Read the model definition and answer for the solid it produces. Units are mm, in the model's axes. Face numbers are marked on the shaded views. A direction names the side the tool comes from. Round coordinates to 2 decimals unless told otherwise and drop trailing zeros. Write each loop counter-clockwise with the first axis right and the second up, starting at its lowest first coordinate (ties: lowest second). Pieces come first, ordered by that corner, then holes. Notation, with made-up numbers: (42.5, 56) - (63.5, 56) arc R14 cw to (63.5, 79) - close; hole circle Ø2 at (42.5, 7.5). An arc over 180 degrees is marked (long way). One line per item, written item: value. Start each with the question number.
(1) Find the intervals of material crossed by L1, parallel to Y at x = -1.25, z = 8.25; L2, parallel to X at y = -1, z = 4.75; L3, parallel to Z at x = 4, y = 1.5, in increasing order.
(2) The mould has two halves that part along Z. Classify the marked faces 1, 2 and 3: +Z half, -Z half, draft (parallel to the pull), parting line (faces both ways), or undercut.
(3) Flat-ended cylindrical pins translate along their axes: pin 1 Ø1.1 at (x, y) = (0.5, 3.5) entering from -Z; pin 2 Ø2.5 at (x, z) = (3.5, 3) entering from -Y; pin 3 Ø2.5 at (x, z) = (0.5, -4.5) entering from +Y. Find the tip coordinate at first contact, or state that the pin passes through.
(4) A cutting plane is placed at A-A, the plane z = -4.5. Determine the outline of the cut face in (x, y), plus the area to 3 significant figures.
(5) A cutting plane is placed at C-C, the plane z = -0.5. Determine the outline of the cut face in (x, y), plus the area to 3 significant figures.
(6) For the marked faces 4 and 5, determine the directions among +Z, -Z, +X, -X, +Y, -Y from which every point of the face is accessible in a straight line to the end or side of a thin tool.
(7) A cutting plane is placed at B-B, the plane y = -2. Determine the outline of the cut face in (x, z), plus the area to 3 significant figures.
from build123d import *

# Parameters (mm, degrees)
F0_W      = 16.9
F0_H      = 26
F1_DEPTH  = 6
F4_DEPTH  = 8
F7_DEPTH  = 13
F13_R     = 1.0372867361
F14_DEPTH = 3
F16_DEPTH = 12


# Not quite as in the source:
# - the arcs of a loft's sections are written as splines that run evenly, so that the points pair up as in the source's solid


with BuildPart() as f1:
    # F0 (on Right) → F1 (new body, symmetric)
    with BuildSketch(Plane.YZ):
        Rectangle(F0_W, F0_H)
    extrude(amount=F1_DEPTH, both=True)

    # F3 (on offset) → F4 (cut)
    with BuildSketch(Plane.YZ.offset(6)):
        with BuildLine():
            Line((0, -13.1401689723), (0, 0))
            Line((0, 0), (0, 8.9160166681))
            ThreePointArc((0, 8.9160166681), (-3.6351196468, 12.5511363149), (-7.2702392936, 8.9160166681))
            Line((-7.2702392936, 8.9160166681), (-7.2702392936, 0))
            Line((-7.2702392936, 0), (-7.2702392936, -13.1401689723))
            Line((-7.2702392936, -13.1401689723), (0, -13.1401689723))
        make_face()
    extrude(amount=-F4_DEPTH, mode=Mode.SUBTRACT)

    # F6 (on offset) → F7 (cut)
    with BuildSketch(Plane.XY.offset(-13)):
        with BuildLine():
            Line((0, 1.0551682208), (6, 1.0551682208))
            Line((6, 1.0551682208), (6, 4.8324568197))
            Line((6, 4.8324568197), (0, 4.8324568197))
            ThreePointArc((0, 4.8324568197), (-1.8886442995, 2.9438125202), (0, 1.0551682208))
        make_face()
    extrude(amount=F7_DEPTH, mode=Mode.SUBTRACT)

    # F10 (on offset) → F11 section 0
    with BuildSketch(Plane.XY.offset(13)):
        with BuildLine():
            add(Edge.make_bspline(
                [(4.3429478235, 3.9498277403), (4.3273258404, 4.518318281), (4.1986746967, 5.0834789619), (3.734705213, 6.1219559637), (3.3995694252, 6.5948636881), (2.5735095721, 7.3767379005), (2.0829105259, 7.6853967543), (1.0205204277, 8.0916349162), (0.4491473807, 8.1890543869), (-0.6878337007, 8.1578104207), (-1.2529943817, 8.0291592769), (-2.2914713834, 7.5651897932), (-2.7643791079, 7.2300540055), (-3.5462533203, 6.4039941523), (-3.8549121741, 5.9133951062), (-4.261150336, 4.8510050079), (-4.3585698066, 4.279631961), (-4.3429478235, 3.7111414202)],
                knots=[0, 0, 0, 0, 0.125, 0.125, 0.25, 0.25, 0.375, 0.375, 0.5, 0.5, 0.625, 0.625, 0.75, 0.75, 0.875, 0.875, 1, 1, 1, 1], degree=3))
            add(Edge.make_bspline(
                [(-4.3429478235, 3.7111414202), (-4.3273258404, 3.1426508795), (-4.1986746967, 2.5774901986), (-3.734705213, 1.5390131968), (-3.3995694252, 1.0661054724), (-2.5735095721, 0.28423126), (-2.0829105259, -0.0244275938), (-1.0205204277, -0.4306657557), (-0.4491473807, -0.5280852264), (0.6878337007, -0.4968412602), (1.2529943817, -0.3681901164), (2.2914713834, 0.0957793673), (2.7643791079, 0.430915155), (3.5462533203, 1.2569750082), (3.8549121741, 1.7475740543), (4.261150336, 2.8099641525), (4.3585698066, 3.3813371995), (4.3429478235, 3.9498277403)],
                knots=[0, 0, 0, 0, 0.125, 0.125, 0.25, 0.25, 0.375, 0.375, 0.5, 0.5, 0.625, 0.625, 0.75, 0.75, 0.875, 0.875, 1, 1, 1, 1], degree=3))
        make_face()
    # F8 (on Top) → F11 section 1
    with BuildSketch(Plane.XY):
        with BuildLine():
            Line((6, 1.9599355292), (6, 3.9953631349))
            add(Edge.make_bspline(
                [(6, 3.9953631349), (5.8728482854, 4.0351535262), (5.7381950052, 4.0508266131), (5.4724119576, 4.0317817528), (5.3413690344, 3.9970700285), (5.1010102922, 3.8820439003), (4.9917730101, 3.8017670809), (4.8102123375, 3.6067310401), (4.7379482715, 3.4920355462), (4.640395332, 3.2440703086), (4.6151383336, 3.110881587), (4.6151383336, 2.844417077), (4.640395332, 2.7112283554), (4.7379482715, 2.4632631178), (4.8102123375, 2.348567624), (4.9917730101, 2.1535315831), (5.1010102922, 2.0732547638), (5.3413690344, 1.9582286356), (5.4724119576, 1.9235169113), (5.7381950052, 1.904472051), (5.8728482854, 1.9201451378), (6, 1.9599355292)],
                knots=[0, 0, 0, 0, 0.1, 0.1, 0.2, 0.2, 0.3, 0.3, 0.4, 0.4, 0.5, 0.5, 0.6, 0.6, 0.7, 0.7, 0.8, 0.8, 0.9, 0.9, 1, 1, 1, 1], degree=3))
        make_face()
    loft(ruled=True, mode=Mode.SUBTRACT)

    # F13 (on offset) → F14 (cut)
    with BuildSketch(Plane.YZ.offset(-2)):
        with Locations((-4.3216282502, 0)):
            Circle(F13_R)
    extrude(amount=-F14_DEPTH, mode=Mode.SUBTRACT)

    # F15 (on offset) → F16 (cut)
    with BuildSketch(Plane.YZ.offset(6)):
        with BuildLine():
            Line((8.45, -5.9837657027), (8.45, 5.8088130318))
            ThreePointArc((8.45, 5.8088130318), (7.3449803731, -0.0874763355), (8.45, -5.9837657027))
        make_face()
        with BuildLine():
            Line((-8.45, 4.3591358699), (-8.45, -5.9991455637))
            ThreePointArc((-8.45, -5.9991455637), (-7.6726197795, -0.8200048469), (-8.45, 4.3591358699))
        make_face()
    extrude(amount=-F16_DEPTH, mode=Mode.SUBTRACT)


solid = f1.part
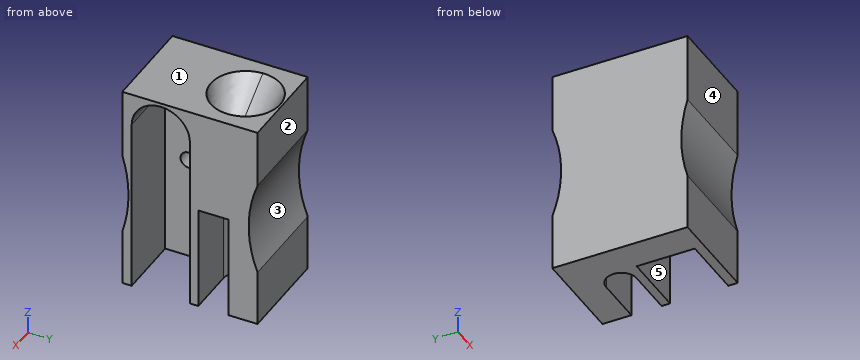
Here are the results:
1. L1: -8.45 to -7.27, 0 to 8.45
1. L2: -6 to -2
1. L3: 0 to 13
2. face 1: +Z half
2. face 2: draft
2. face 3: undercut
3. pin 1: z = 0
3. pin 2: y = -8.42
3. pin 3: y = 8.36
4. outline: (-6, -8.06) - (6, -8.06) - (6, -7.27) - (-2, -7.27) - (-2, 0) - (6, 0) - (6, 1.06) - (0, 1.06) arc R1.89 cw to (0, 4.83) - (6, 4.83) - (6, 7.95) - (-6, 7.95) - close
4. area: 106 mm²
5. outline: (-6, -7.68) - (6, -7.68) - (6, -7.27) - (-2, -7.27) - (-2, -5.23) - (-5, -5.23) - (-5, -3.41) - (-2, -3.41) - (-2, 0) - (6, 0) - (6, 1.06) - (0, 1.06) arc R1.89 cw to (0, 4.83) - (6, 4.83) - (6, 7.35) - (-6, 7.35) - close
5. area: 88.4 mm²
6. face 4: +Z, -Z, +X, -X, -Y
6. face 5: -Z, +X
7. outline: (-6, -13) - (-2, -13) - (-2, 12.16) - (6, 12.16) - (6, 13) - (-6, 13) - close
7. area: 111 mm²
